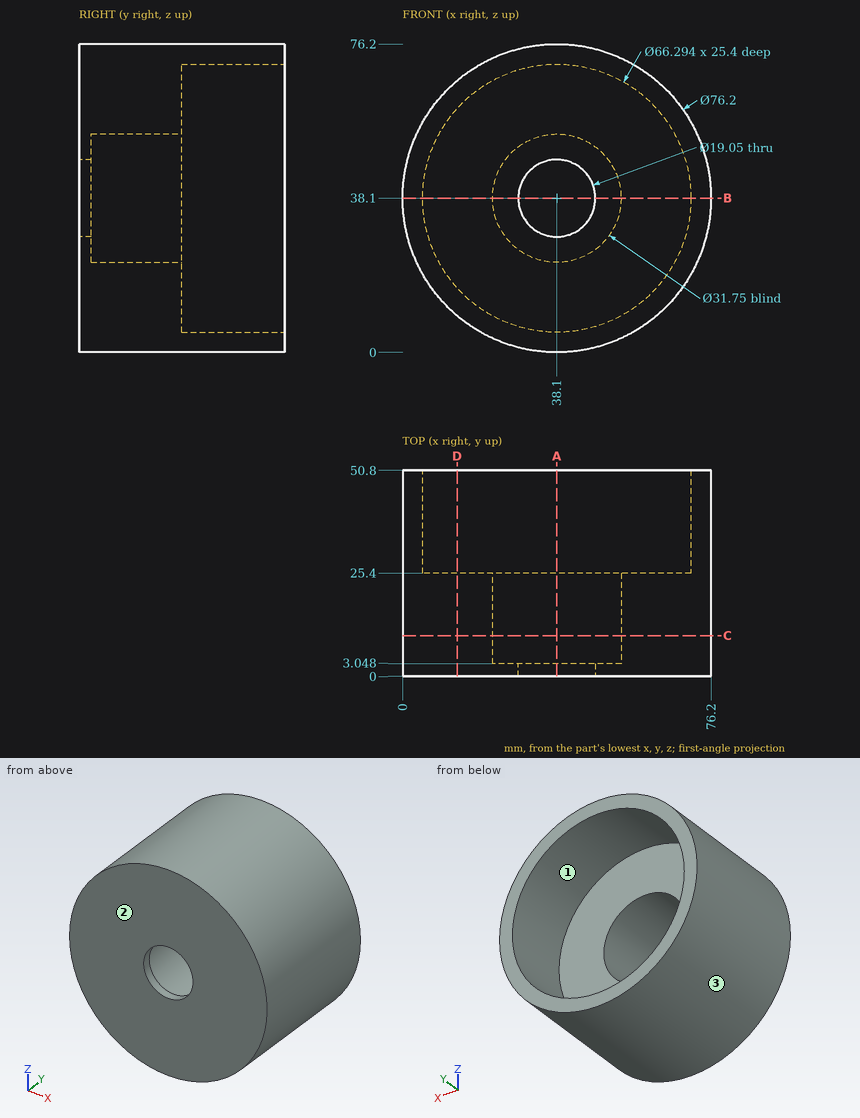
The figure shows three views and two pictorial views of one solid part (mm, origin at its lowest corner). Answer the questions. Coordinates: 2 decimals unless noted, no trailing zeros. Write each loop counter-clockwise with the first axis right and the second up, starting at its lowest first coordinate (ties: lowest second). Pieces come first, ordered by that corner, then holes. Notation, with made-up numbers: (26.25, 28) -> (38.25, 28) arc R19 cw to (38.25, 60) -> close; hole circle Ø2 at (-4, 27.5). An arc over 180 degrees is marked (long way). Return JSON: item names as keys, results as strings.
1. Each of these flat-tipped pins is pushed along its axis until it touches: P1, Ø8, axis at y = 42.5, z = 8.5, coming from the +X side; P2, Ø5, axis at x = 59, z = 27.5, coming from the +Y side; P3, Ø1, axis at x = 49, y = 38, coming from the -Z side. Where does it stop, or does it pass through?
Found:
{"P1": "x = 66.32", "P2": "y = 25.4", "P3": "z = 1.45"}
2. Determine the mould class of the marked faces 1, 2 and 3 for opening direction Z: pulls with the +Z half, pulls with the -Z half, needs draft (parallel to the pull), parting line crosses it, or undercut.
Found:
{"face 1": "undercut", "face 2": "needs draft", "face 3": "parting line crosses it"}
3. Find the intervals of material crossed by line 1 along X through (y, z) = (18, 38); line 2 along Z through (x, y) = (38.1, 15.25) (3 decimals); line 3 along X through (y, z) = (1.3, 38.1) (3 decimals), in increasing order. Write a range as from..to.
Found:
{"line 1": "0..22.23, 53.97..76.2", "line 2": "0..22.225, 53.975..76.2", "line 3": "0..28.575, 47.625..76.2"}
4. A cutting plane is placed at D-D (x = 13.5). Determine the outline of the cut face in (y, z).
Found:
{"outline": "(0, 9.01) -> (50.8, 9.01) -> (50.8, 15.88) -> (25.4, 15.88) -> (25.4, 60.32) -> (50.8, 60.32) -> (50.8, 67.19) -> (0, 67.19) -> close"}
5. A cutting plane is placed at B-B (z = 38.1). Determine the outline of the cut face in (x, y) (3 decimals), and give its area (3 significant figures).
Found:
{"outline": "(0, 0) -> (28.575, 0) -> (28.575, 3.048) -> (22.225, 3.048) -> (22.225, 25.4) -> (4.953, 25.4) -> (4.953, 50.8) -> (0, 50.8) -> close; (47.625, 0) -> (76.2, 0) -> (76.2, 50.8) -> (71.247, 50.8) -> (71.247, 25.4) -> (53.975, 25.4) -> (53.975, 3.048) -> (47.625, 3.048) -> close", "area": "1,420 mm2"}
6. A cutting plane is placed at A-A (x = 38.1). Determine the outline of the cut face in (y, z) (3 decimals).
Found:
{"outline": "(0, 0) -> (50.8, 0) -> (50.8, 4.953) -> (25.4, 4.953) -> (25.4, 22.225) -> (3.048, 22.225) -> (3.048, 28.575) -> (0, 28.575) -> close; (0, 47.625) -> (3.048, 47.625) -> (3.048, 53.975) -> (25.4, 53.975) -> (25.4, 71.247) -> (50.8, 71.247) -> (50.8, 76.2) -> (0, 76.2) -> close"}
7. A cutting plane is placed at C-C (y = 10). Determine the outline of the cut face in (x, z) (3 decimals).
Found:
{"outline": "circle Ø76.2 at (38.1, 38.1); hole circle Ø31.75 at (38.1, 38.1)"}
